```python
from build123d import *
from build123d.topology import SkipClean

# Parameters (mm, degrees)
SKETCH1_R           = 45.85
SKETCH1_R_2         = 7.5
SKETCH1_R_3         = 1.5635
BOSS_EXTRUDE1_DEPTH = 4.7625
SKETCH1_6_R         = 1.8125
SKETCH1_6_R_2       = 3
CUT_EXTRUDE1_DEPTH  = 2.5
BOSS_EXTRUDE2_START = 12.15
SKETCH1_7_R         = 45.85
SKETCH1_7_R_2       = 1.5635
BOSS_EXTRUDE2_DEPTH = 12.15
SKETCH2_R           = 1.925
CUT_EXTRUDE2_DEPTH  = 4
CUT_EXTRUDE3_START  = -3.9625
SKETCH1_8_R         = 8.25
SKETCH1_8_R_2       = 7.5
CUT_EXTRUDE3_DEPTH  = 0.8


with BuildPart() as part:
    # Sketch1 → Boss-Extrude1 (new body)
    with BuildSketch(Plane(origin=(0, 0, 0), x_dir=(1, 0, 0), z_dir=(0, 1, 0))):
        with Locations(Location((0, 0, 0), (0, 0, 270))):
            Circle(SKETCH1_R)
        with Locations(Location((0, 0, 0), (0, 0, 270))):
            Circle(SKETCH1_R_2, mode=Mode.SUBTRACT)
        with Locations(Location((-42.5, 0, 0), (0, 0, 270))):
            Circle(SKETCH1_R_3, mode=Mode.SUBTRACT)
        with Locations(Location((0, 42.5, 0), (0, 0, 270))):
            Circle(SKETCH1_R_3, mode=Mode.SUBTRACT)
        with Locations(Location((42.5, 0, 0), (0, 0, 270))):
            Circle(SKETCH1_R_3, mode=Mode.SUBTRACT)
        with Locations(Location((0, -42.5, 0), (0, 0, 270))):
            Circle(SKETCH1_R_3, mode=Mode.SUBTRACT)
    extrude(amount=-BOSS_EXTRUDE1_DEPTH)

    # Sketch1_6 → Cut-Extrude1 (cut)
    with BuildSketch(Plane(origin=(0, 0, 0), x_dir=(1, 0, 0), z_dir=(0, 1, 0))):
        with Locations(Location((-30.5, 0, 0), (0, 0, 270))):
            Circle(SKETCH1_6_R)
        with Locations(Location((-21.566756826, 21.566756826, 0), (0, 0, 270))):
            Circle(SKETCH1_6_R)
        with Locations(Location((0, 30.5, 0), (0, 0, 270))):
            Circle(SKETCH1_6_R)
        with Locations(Location((21.566756826, 21.566756826, 0), (0, 0, 270))):
            Circle(SKETCH1_6_R)
        with Locations(Location((30.5, 0, 0), (0, 0, 270))):
            Circle(SKETCH1_6_R)
        with Locations(Location((21.566756826, -21.566756826, 0), (0, 0, 270))):
            Circle(SKETCH1_6_R)
        with Locations(Location((0, -30.5, 0), (0, 0, 270))):
            Circle(SKETCH1_6_R)
        with Locations(Location((-21.566756826, -21.566756826, 0), (0, 0, 270))):
            Circle(SKETCH1_6_R)
        with Locations(Location((-36.680535028, 7.796688406, 0), (0, 0, 270))):
            Circle(SKETCH1_6_R_2)
        with Locations(Location((-36.680535028, -7.796688406, 0), (0, 0, 270))):
            Circle(SKETCH1_6_R_2)
        with Locations(Location((-30.338137289, 22.041946961, 0), (0, 0, 270))):
            Circle(SKETCH1_6_R_2)
        with Locations(Location((-30.338137289, -22.041946961, 0), (0, 0, 270))):
            Circle(SKETCH1_6_R_2)
        with Locations(Location((-18.75, -32.475952642, 0), (0, 0, 270))):
            Circle(SKETCH1_6_R_2)
        with Locations(Location((-3.919817373, -37.294571076, 0), (0, 0, 270))):
            Circle(SKETCH1_6_R_2)
        with Locations(Location((11.588137289, -35.664619361, 0), (0, 0, 270))):
            Circle(SKETCH1_6_R_2)
        with Locations(Location((25.092397738, -27.867930955, 0), (0, 0, 270))):
            Circle(SKETCH1_6_R_2)
        with Locations(Location((34.257954662, -15.252624115, 0), (0, 0, 270))):
            Circle(SKETCH1_6_R_2)
        with Locations(Location((37.5, 0, 0), (0, 0, 270))):
            Circle(SKETCH1_6_R_2)
        with Locations(Location((34.257954662, 15.252624115, 0), (0, 0, 270))):
            Circle(SKETCH1_6_R_2)
        with Locations(Location((25.092397738, 27.867930955, 0), (0, 0, 270))):
            Circle(SKETCH1_6_R_2)
        with Locations(Location((11.588137289, 35.664619361, 0), (0, 0, 270))):
            Circle(SKETCH1_6_R_2)
        with Locations(Location((-3.919817373, 37.294571076, 0), (0, 0, 270))):
            Circle(SKETCH1_6_R_2)
        with Locations(Location((-18.75, 32.475952642, 0), (0, 0, 270))):
            Circle(SKETCH1_6_R_2)
    extrude(amount=-CUT_EXTRUDE1_DEPTH, mode=Mode.SUBTRACT)

    # Sketch1_7 → Boss-Extrude2 (add)
    with SkipClean():  # the faces are left unmerged after this step: merging them gives an invalid solid
        with BuildSketch(Plane(origin=(0, 0, 0), x_dir=(1, 0, 0), z_dir=(0, 1, 0)).offset(BOSS_EXTRUDE2_START)):
            with Locations(Location((0, 0, 0), (0, 0, 270))):
                Circle(SKETCH1_7_R)
            with Locations(Location((0, -42.5, 0), (0, 0, 270))):
                Circle(SKETCH1_7_R_2, mode=Mode.SUBTRACT)
            with Locations(Location((-42.5, 0, 0), (0, 0, 270))):
                Circle(SKETCH1_7_R_2, mode=Mode.SUBTRACT)
            with Locations(Location((42.5, 0, 0), (0, 0, 270))):
                Circle(SKETCH1_7_R_2, mode=Mode.SUBTRACT)
            with BuildLine():
                ThreePointArc((36.883333333, 2.935936345), (39.39076704, 2.32916294), (40.5, 0))
                ThreePointArc((40.5, 0), (39.39076704, -2.32916294), (36.883333333, -2.935936345))
                ThreePointArc((36.883333333, -2.935936345), (36.191461227, -7.69273256), (34.888754523, -12.319691873))
                ThreePointArc((34.888754523, -12.319691873), (36.59166411, -13.367471546), (37.257954662, -15.252624115))
                ThreePointArc((37.257954662, -15.252624115), (35.6231437, -17.924001829), (32.500448736, -17.683914497))
                ThreePointArc((32.500448736, -17.683914497), (29.933628792, -21.748054335), (26.861593101, -25.445133446))
                ThreePointArc((26.861593101, -25.445133446), (27.767055295, -26.50917897), (28.092397738, -27.867930955))
                ThreePointArc((28.092397738, -27.867930955), (25.872343464, -30.764771418), (22.497941295, -29.37418318))
                ThreePointArc((22.497941295, -29.37418318), (18.5, -32.04293994), (14.189818202, -34.170880284))
                ThreePointArc((14.189818202, -34.170880284), (14.486847583, -34.891651942), (14.588137289, -35.664619361))
                ThreePointArc((14.588137289, -35.664619361), (11.748752331, -38.660316744), (8.605335417, -35.985388734))
                ThreePointArc((8.605335417, -35.985388734), (3.867553141, -36.797310129), (-0.935505175, -36.988171489))
                ThreePointArc((-0.935505175, -36.988171489), (-0.92374189, -37.141170608), (-0.919817373, -37.294571076))
                ThreePointArc((-0.919817373, -37.294571076), (-4.385552663, -40.258199029), (-6.775211132, -36.37439366))
                ThreePointArc((-6.775211132, -36.37439366), (-11.433628792, -35.189091103), (-15.899071208, -33.409871815))
                ThreePointArc((-15.899071208, -33.409871815), (-20.25, -35.074028853), (-20.984262125, -30.47393547))
                ThreePointArc((-20.984262125, -30.47393547), (-24.757832435, -27.496358543), (-28.113543391, -24.054701786))
                ThreePointArc((-28.113543391, -24.054701786), (-32.765188272, -23.805302718), (-31.564943561, -19.304256991))
                ThreePointArc((-31.564943561, -19.304256991), (-33.801181933, -15.049255794), (-35.466928517, -10.540255288))
                ThreePointArc((-35.466928517, -10.540255288), (-39.61497783, -8.420423478), (-36.687759497, -4.796697105))
                ThreePointArc((-36.687759497, -4.796697105), (-37, 0), (-36.687759497, 4.796697105))
                ThreePointArc((-36.687759497, 4.796697105), (-39.61497783, 8.420423478), (-35.466928517, 10.540255288))
                ThreePointArc((-35.466928517, 10.540255288), (-33.801181933, 15.049255794), (-31.564943561, 19.304256991))
                ThreePointArc((-31.564943561, 19.304256991), (-32.765188272, 23.805302718), (-28.113543391, 24.054701786))
                ThreePointArc((-28.113543391, 24.054701786), (-24.757832435, 27.496358543), (-20.984262125, 30.47393547))
                ThreePointArc((-20.984262125, 30.47393547), (-20.25, 35.074028853), (-15.899071208, 33.409871815))
                ThreePointArc((-15.899071208, 33.409871815), (-11.433628792, 35.189091103), (-6.775211132, 36.37439366))
                ThreePointArc((-6.775211132, 36.37439366), (-4.385552663, 40.258199029), (-0.919817373, 37.294571076))
                ThreePointArc((-0.919817373, 37.294571076), (-0.92374189, 37.141170608), (-0.935505175, 36.988171489))
                ThreePointArc((-0.935505175, 36.988171489), (3.867553141, 36.797310129), (8.605335417, 35.985388734))
                ThreePointArc((8.605335417, 35.985388734), (11.748752331, 38.660316744), (14.588137289, 35.664619361))
                ThreePointArc((14.588137289, 35.664619361), (14.486847583, 34.891651942), (14.189818202, 34.170880284))
                ThreePointArc((14.189818202, 34.170880284), (18.5, 32.04293994), (22.497941295, 29.37418318))
                ThreePointArc((22.497941295, 29.37418318), (25.872343464, 30.764771418), (28.092397738, 27.867930955))
                ThreePointArc((28.092397738, 27.867930955), (27.767055295, 26.50917897), (26.861593101, 25.445133446))
                ThreePointArc((26.861593101, 25.445133446), (29.933628792, 21.748054335), (32.500448736, 17.683914497))
                ThreePointArc((32.500448736, 17.683914497), (35.6231437, 17.924001829), (37.257954662, 15.252624115))
                ThreePointArc((37.257954662, 15.252624115), (36.59166411, 13.367471546), (34.888754523, 12.319691873))
                ThreePointArc((34.888754523, 12.319691873), (36.191461227, 7.69273256), (36.883333333, 2.935936345))
            make_face(mode=Mode.SUBTRACT)
            with Locations(Location((0, 42.5, 0), (0, 0, 270))):
                Circle(SKETCH1_7_R_2, mode=Mode.SUBTRACT)
        extrude(amount=-BOSS_EXTRUDE2_DEPTH)

    # Sketch2 → Cut-Extrude2 (cut)
    with SkipClean():  # the faces are left unmerged after this step: merging them gives an invalid solid
        with BuildSketch(Plane(origin=(0, 12.15, 0), x_dir=(1, 0, 0), z_dir=(0, 1, 0))):
            with Locations(Location((-42.5, 0, 0), (0, 0, 270))):
                Circle(SKETCH2_R)
            with Locations(Location((0, 42.5, 0), (0, 0, 270))):
                Circle(SKETCH2_R)
            with Locations(Location((42.5, 0, 0), (0, 0, 270))):
                Circle(SKETCH2_R)
            with Locations(Location((0, -42.5, 0), (0, 0, 270))):
                Circle(SKETCH2_R)
        extrude(amount=-CUT_EXTRUDE2_DEPTH, mode=Mode.SUBTRACT)

    # Sketch1_8 → Cut-Extrude3 (cut)
    with SkipClean():  # the faces are left unmerged after this step: merging them gives an invalid solid
        with BuildSketch(Plane(origin=(0, 0, 0), x_dir=(1, 0, 0), z_dir=(0, 1, 0)).offset(CUT_EXTRUDE3_START)):
            with Locations(Location((0, 0, 0), (0, 0, 270))):
                Circle(SKETCH1_8_R)
            with Locations(Location((0, 0, 0), (0, 0, 270))):
                Circle(SKETCH1_8_R_2, mode=Mode.SUBTRACT)
        extrude(amount=-CUT_EXTRUDE3_DEPTH, mode=Mode.SUBTRACT)


solid = part.part
```
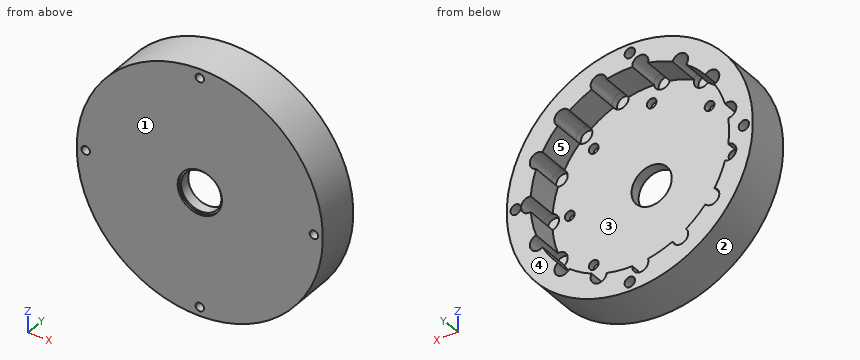
Model file for the job. Use its own axes, mm. Face numbers are marked on the shaded views. A direction names the side the tool comes from. Coordinates: 2 decimals unless noted, no trailing zeros. Order: outer loops, then holes, each group sorted by start corner. A loop starts at its lowest first (then second) coordinate and runs counter-clockwise, first axis right, second up. Notation, with made-up numbers: (26.25, 75) - (84.25, 75) arc R17 ccw to (84.25, 95) - close; hole circle Ø9 at (15, 10). An arc over 180 degrees is marked (long way). Return JSON: item names as keys, results as strings. Group by question number.
1) Mould opens along Z. For the marked faces 1, 2 and 3 say: released by +Z, released by -Z, zero draft, split by the parting line, or undercut.
2) Saw through at C-C, the plane y = 3.75. Count the separate pieces of the cut face and the enclosed holes in it, plus the area to 3 significant figures.
3) Probe line 1 (X direction, y = -4.25, z = 0); line 2 (Z direction, x = -38.5, y = 1.25); line 3 (X direction, y = 1.75, z = -18). List the from-to ranges inside material, lowest first. Write a range as from..to.
4) Tool access for the marked faces 4 and 5: list every direction of +Z, -Z, +X, -X, +Y, -Y with a clear straight run to the whole face (end or side of a thin tool).
5) Saw through at D-D, the plane x = -17. Write the cut outline in (y, z).
6) Flat gauge pins, fed straight in: P1, Ø6, axis at x = 30.5, z = 0, coming from the +Y side; P2, Ø5, axis at y = 3, z = 2.5, coming from the +X side; P3, Ø4, axis at x = -0.5, z = 43, coming from the +Y side; P4, Ø2, axis at y = 8, z = -0.5, coming from the -X side. Where does each tip first touch, or does it go through?
Values found:
{
 "1": {"face 1": "zero draft", "face 2": "split by the parting line", "face 3": "undercut"},
 "2": {"separate pieces": "1", "enclosed holes": "5", "area": "2,010 mm²"},
 "3": {"line 1": "x = -45.85..-44.06, -40.94..-8.25, 8.25..40.94, 44.06..45.85", "line 2": "z = -24.9..-10.18, -5.41..5.41, 10.18..24.9", "line 3": "x = -42.17..-32.33, 32.33..33.05, 35.46..42.17"},
 "4": {"face 4": "+Z, -Z, +X, -X, +Y", "face 5": "+Y"},
 "5": {"outline": "(-4.76, -42.58) - (12.15, -42.58) - (12.15, -34.91) - (-2.5, -34.91) - (-2.5, -30.04) - (0, -30.04) - (0, 30.04) - (-2.5, 30.04) - (-2.5, 34.91) - (12.15, 34.91) - (12.15, 42.58) - (-4.76, 42.58) - close"},
 "6": {"P1": "stops at y = 0", "P2": "stops at x = 45.85", "P3": "stops at y = 12.15", "P4": "stops at x = -45.85"}
}
